Input: part model. Units: mm. Frame: model coordinates. A direction names the side the tool comes from. Round coordinates to 2 decimals unless told otherwise and drop trailing zeros. One line per question, with ' | ' between items. Start each with the question number.
Item 1: Draft query along Y for faces 1 (the face through (0, -24.3, 7.6)), 2 (the face through (2.5, -19.1, -11.2)), 3 (the face through (11.9, -1.43, 0.32)). Return one class per face: pulls with the +Y half, pulls with the -Y half, needs draft (parallel to the pull), parting line crosses it, or undercut.
Item 2: Material intervals for line 1 along Y through (x, z) = (7.75, -8); line 2 along X through (y, z) = (-19, -10.5); line 3 along Y through (x, z) = (-11, 0), sorted ascending.
Item 3: Set-up query: faces 4 (the face through (2.15, -3.13, 7.92)), 5 (the face through (0, -4, 5)), 6 (the face through (-2.5, -19.1, -11.2)). Return all of +Z, -Z, +X, -X, +Y, -Y with unobstructed straight access to the full face (end or side cutting, diameter ignored); none if empty.
Item 4: First-contact query: pin 1 (4 mm diameter, centred on x = 6, z = 3, fed in from +Y); pin 2 (12 mm diameter, centred on y = -25, z = 3.5, fed in from -X); pin 3 (12 mm diameter, centred on x = 10, y = -12, fed in from +Z); pin 4 (5 mm diameter, centred on y = -25, z = -10, fed in from +X). Flat tips, straight axial feed; report the tip coordinate or a pass-through.
```python
from build123d import *

# Parameters (mm, degrees)
F0_W     = 25
F0_H     = 45
F1_DEPTH = 2
F2_W     = 5
F2_H     = 35
F3_DEPTH = 50
F5_DEPTH = 5
F6_R     = 1.99999


# Not quite as in the source:
# - a fillet or chamfer is up to 0.001 mm smaller than in the source, because OpenCascade refuses the exact size


with BuildPart() as f1:
    # F0 (on Front) → F1 (new body)
    with BuildSketch(Plane.XZ):
        Rectangle(F0_W, F0_H)
    extrude(amount=F1_DEPTH)

    # F2 (on face) → F3 (join)
    with BuildSketch(Plane.XZ.offset(2)):
        with Locations((0, 2.5)):
            Rectangle(F2_W, F2_H)
    extrude(amount=F3_DEPTH)

    # F4 (on face) → F5 (cut, through all)
    with BuildSketch(Plane.YZ.offset(2.5)):
        with BuildLine():
            Line((-4, 10), (-2, 20))
            Line((-2, 20), (-52, 20))
            Line((-52, 20), (-52, -15))
            Line((-52, -15), (-14.0000000101, -15))
            ThreePointArc((-14.0000000101, -15), (-23.4927752917, -11.6140956282), (-28.7, -2.9849623113))
            ThreePointArc((-28.7, -2.9849623113), (-28.8931709496, 1.7870252), (-27.5765596133, 6.3778545818))
            ThreePointArc((-27.5765596133, 6.3778545818), (-24.2508239141, 7.5776387537), (-23.0510397422, 4.2519030545))
            ThreePointArc((-23.0510397422, 4.2519030545), (-23.9287806331, 1.1913501333), (-23.8, -1.9899748742))
            ThreePointArc((-23.8, -1.9899748742), (-13, -9.9498743711), (-4, 0))
            Line((-4, 0), (-4, 10))
        make_face()
        with BuildLine():
            Line((-2, -15), (-2, -9))
            ThreePointArc((-2, -9), (-7.291796072, -13.4164078673), (-14.0000000101, -15))
            Line((-14.0000000101, -15), (-2, -15))
        make_face()
    extrude(amount=-F5_DEPTH, mode=Mode.SUBTRACT)

    # F6 (radius 2 in the source; OpenCascade refuses exactly that, so slightly less here)
    f6_edges = [f1.edges().sort_by_distance(p)[0] for p in [
        (2.5, -24.250824, 7.577639),
        (-2.5, -24.250824, 7.577639),
        (0, -2, 22.5),
        (-12.5, -2, 0),
        (0, -2, -22.5),
        (12.5, -2, 0),
    ]]
    fillet(f6_edges, radius=F6_R)


solid = f1.part
```
Return value:
1) face 1: undercut | face 2: needs draft | face 3: pulls with the -Y half
2) line 1: -2 to 0 | line 2: -2.47 to 2.47 | line 3: -1.94 to 0
3) face 4: +Z, +X | face 5: +Z, +X, -X | face 6: +Z, -Z, -X, -Y
4) pin 1: y = 0 | pin 2: x = -2.5 | pin 3: through | pin 4: x = 2.5
